Work out the finished part from the listing and answer in its coordinate system (mm). A direction names the side the tool comes from. Give positions to 0.01 mm unless a question says otherwise; leave off trailing zeros. Loops run counter-clockwise (first coordinate to the right, second up) from the corner with the lowest first, then second, coordinate; pieces in that order, holes last. Notation, with made-up numbers: (81, -31.75) - (121, -31.75) arc R13 ccw to (121, -15.75) - close; hole circle Ø5 at (77, -30.5). An arc over 180 degrees is marked (long way). One line per item, written item: value.
from build123d import *

# Parameters (mm, degrees)
BOSS_EXTRUDE1_DEPTH = 35
SKETCH2_W           = 539.999711362
SKETCH2_H           = 462.5
CUT_EXTRUDE1_DEPTH  = 35
FILLET1_R           = 10


with BuildPart() as part:
    # Sketch1 → Boss-Extrude1 (new body)
    with BuildSketch(Plane(origin=(0, 0, 0), x_dir=(0, 0, -1), z_dir=(1, 0, 0))):
        Polygon((-310.498220641, 250), (289.501486325, 250), (289.501779359, -250), (-310.498220641, -250), align=None)
    extrude(amount=BOSS_EXTRUDE1_DEPTH)

    # Sketch2 → Cut-Extrude1 (cut)
    with BuildSketch(Plane(origin=(35, 0, 0), x_dir=(0, 0, -1), z_dir=(1, 0, 0))):
        with Locations((-10.49836496, 11.25)):
            Rectangle(SKETCH2_W, SKETCH2_H)
    extrude(amount=-CUT_EXTRUDE1_DEPTH, mode=Mode.SUBTRACT)

    # Fillet1
    fillet1_edges = [part.edges().sort_by_distance(p)[0] for p in [
        (17.5, -250, -289.501779359),
        (17.5, -250, 310.498220641),
    ]]
    fillet(fillet1_edges, radius=FILLET1_R)


solid = part.part
1. Find the intervals of material crossed by line 1 along Z through (x, y) = (12, 144.5); line 2 along Y through (x, z) = (2, -187.5), in increasing order.
Output:
line 1: z = -289.5 to -259.5, 280.5 to 310.5
line 2: y = -250 to -220, 242.5 to 250
2. The mould has two halves that part along Z. Classify faces 3 (the flat face through (17, 8, -289.502)), 4 (the flat face through (17, 250, 15)), 5 (the flat face through (18, -220, 14)): released by +Z, released by -Z, zero draft, split by the parting line, or undercut.
Output:
face 3: released by -Z
face 4: zero draft
face 5: undercut
3. Section A-A (x = 20.5) is taken. Write down the section's boundary in (y, z).
Output:
outline: (-250, -279.5) arc R10 ccw to (-240, -289.5) - (250, -289.5) - (250, 310.5) - (-240, 310.5) arc R10 ccw to (-250, 300.5) - close; hole (-220, -259.5) - (242.5, -259.5) - (242.5, 280.5) - (-220, 280.5) - close
4. Section B-B (z = -215) is taken. Write down the section's boundary in (x, y).
Output:
outline: (0, -250) - (35, -250) - (35, -220) - (0, -220) - close; (0, 242.5) - (35, 242.5) - (35, 250) - (0, 250) - close
5. For faces 1 (the flat face through (0, -221, 9)), 2 (the flat face through (18, 8, 280.498)), determine the directions among +Z, -Z, +X, -X, +Y, -Y from which every point of the face is accessible in a straight line to the end or side of a thin tool.
Output:
face 1: +Z, -Z, -X, +Y, -Y
face 2: +X, -X
6. Section C-C (y = 119) is taken. Write down the section's boundary in (x, z), and give its area (3 significant figures).
Output:
outline: (0, -289.5) - (35, -289.5) - (35, -259.5) - (0, -259.5) - close; (0, 280.5) - (35, 280.5) - (35, 310.5) - (0, 310.5) - close
area: 2,100 mm²
